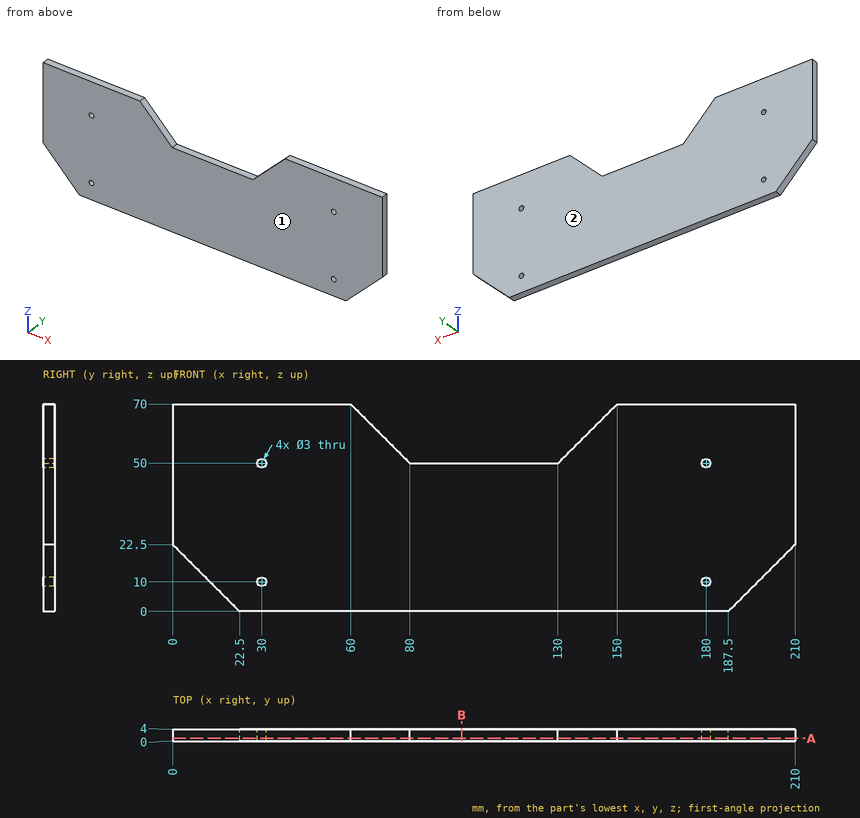
Geometry: see drawing. Coordinates: mm, zero at the bounding-box minimum. Give positions to 0.01 mm unless a question says otherwise; leave off trailing zeros. Write each loop counter-clockwise with the first axis right and the second up, starting at its lowest first coordinate (ties: lowest second). Pieces come first, ordered by that corner, then holes. Notation, with made-up numbers: (36, -12.75) - (81, -12.75) arc R30 ccw to (81, 17.25) - close; hole circle Ø9 at (0.5, 57.5). An arc over 180 degrees is marked (long way). Return JSON: item names as keys, results as strings. Group by question number.
1) Line query: line 1 (Z direction, x = 180, y = 2.3); line 2 (X direction, y = 2.45, z = 10); line 3 (Z direction, x = 118.5, y = 0.6). Output: solid intervals per line, ascending.
2) Section A-A on y = 1. Return the cut outline in (x, z).
3) Mould query, pull axis Y, two halves, no side actions, for the marked faces 1 and 2. Classes: released by +Y, released by -Y, zero draft, split by the parting line, or undercut.
4) Section B-B on x = 97.5. Return the cut outline in (y, z).
Filled in:
{
 "1": {"line 1": "z = 0 to 8.5, 11.5 to 48.5, 51.5 to 70", "line 2": "x = 12.5 to 28.5, 31.5 to 178.5, 181.5 to 197.5", "line 3": "z = 0 to 50"},
 "2": {"outline": "(0, 22.5) - (22.5, 0) - (187.5, 0) - (210, 22.5) - (210, 70) - (150, 70) - (130, 50) - (80, 50) - (60, 70) - (0, 70) - close; hole circle Ø3 at (30, 10); hole circle Ø3 at (30, 50); hole circle Ø3 at (180, 10); hole circle Ø3 at (180, 50)"},
 "3": {"face 1": "released by -Y", "face 2": "released by +Y"},
 "4": {"outline": "(0, 0) - (4, 0) - (4, 50) - (0, 50) - close"}
}
